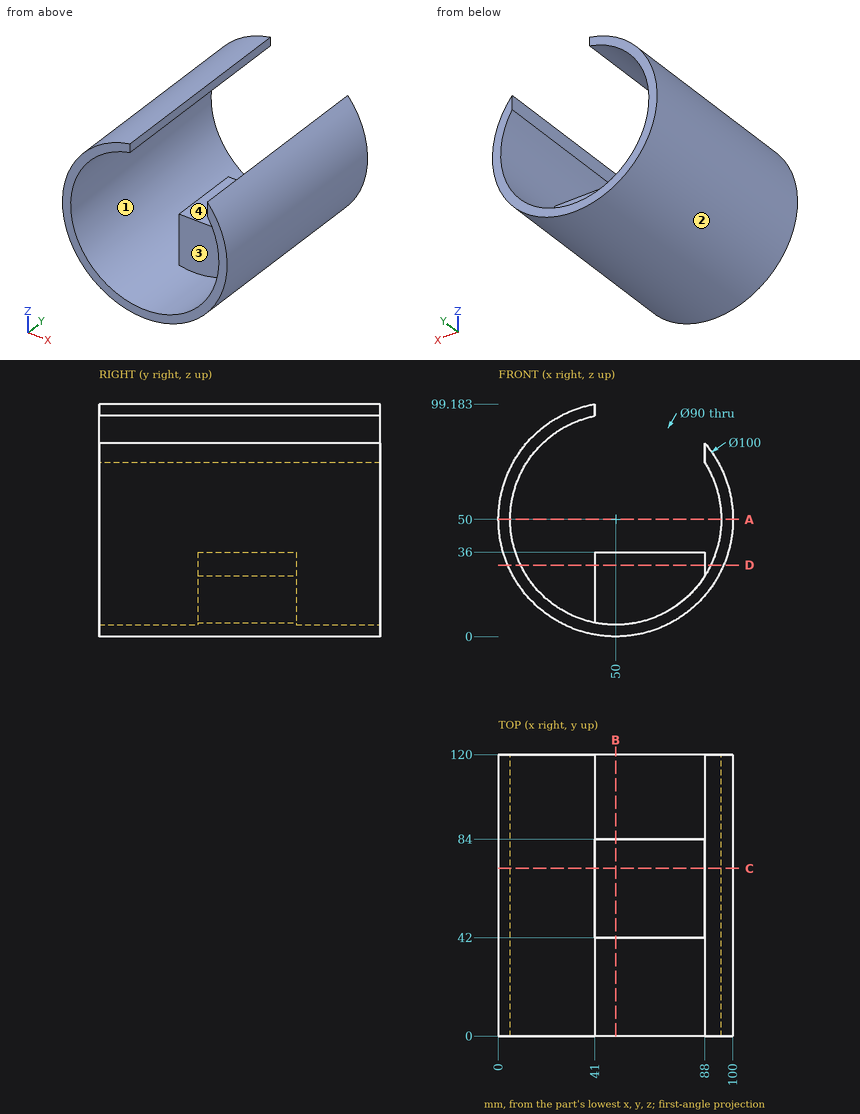
Here's the drawing with two shaded views (mm, measured from the low corner). I have some questions. A direction names the side the tool comes from. Round coordinates to 2 decimals unless told otherwise and drop trailing zeros. Loops run counter-clockwise (first coordinate to the right, second up) from the corner with the lowest first, then second, coordinate; pieces in that order, holes last. Notation, with made-up numbers: (49, 57) -> (67, 57) arc R17 ccw to (67, 62) -> close; hole circle Ø7 at (7.5, 78). An arc over 180 degrees is marked (long way). Answer as CSV lines item,"result". Start each with the question number.
1. For the marked faces 3 and 4, which set-ups out of +Z, -Z, +X, -X, +Y, -Y let a thin tool reach every point of the face, with its end or its side?
2. I need wall thicknesses on probe 1 along X at (y, z) = (93, 50); probe 2 along X at (y, z) = (53, 26.5) (1 decimal); probe 3 along Y at (x, z) = (45, 27). Which ranges of each line are inside material? Lowest first, please. Write a range as from..to.
3. I'm going to push flat-ended pins straight in: P1, Ø2, axis at x = 38, y = 27.5, coming from the +Z side (1 decimal); P2, Ø1.5, axis at y = 83.5, z = 96, coming from the +X side; P3, Ø6, axis at x = 20, y = 17, coming from the -Z side. Where does each tip first touch, or does it pass through?
4. If we mould it in two halves opening along X, with no side actions, what happens to the marked faces 1 and 2? For each: pulls with the +X half, pulls with the -X half, needs draft (parallel to the pull), parting line crosses it, or undercut.
5. Imagine slicing it at A-A on z = 50. Write out the boundary of the cut face in (x, y).
6. Imagine slicing it at C-C on y = 71.5. Write out the boundary of the cut face in (x, z).
7. Imagine slicing it at B-B on x = 50. Write out the boundary of the cut face in (y, z).
8. Imagine slicing it at D-D on z = 30.5. Write out the boundary of the cut face in (x, y) (1 decimal).
Solution:
1,face 3,"+Z, -Y"
1,face 4,"+Z, +Y, -Y"
2,probe 1,"0..5, 95..100"
2,probe 2,"5.9..11.6, 41..88, 88.4..94.1"
2,probe 3,"42..84"
3,P1,"z = 98.8"
3,P2,"x = 41"
3,P3,"z = 7.92"
4,face 1,"undercut"
4,face 2,"parting line crosses it"
5,outline,"(0, 0) -> (5, 0) -> (5, 120) -> (0, 120) -> close; (95, 0) -> (100, 0) -> (100, 120) -> (95, 120) -> close"
6,outline,"(41, 5.91) arc R45 cw to (41, 94.09) -> (41, 99.18) arc R50 ccw (long way) to (88, 82.5) -> (88, 74.1) arc R45 cw to (88, 25.9) -> (88, 36) -> (41, 36) -> close"
7,outline,"(0, 0) -> (120, 0) -> (120, 5) -> (84, 5) -> (84, 36) -> (42, 36) -> (42, 5) -> (0, 5) -> close"
8,outline,"(4, 0) -> (9.4, 0) -> (9.4, 120) -> (4, 120) -> close; (41, 42) -> (88, 42) -> (88, 84) -> (41, 84) -> close; (90.6, 0) -> (96, 0) -> (96, 120) -> (90.6, 120) -> close"
